Autodesk Inventor part; units mm, degrees
ref_plane "XZ Plane" through (0, 0, 0) normal (0, 1, 0) x (-1, 0, 0)
ref_plane "XY Plane" through (0, 0, 0) normal (0, 0, 1) x (1, 0, 0)
ref_plane "РабПлоскость1" through (0, 0, 0) normal (0, 0, 1) x (1, 0, 0)
sketch "Эскиз1" plane through (0, 0, 0) normal (0, 0, 1) x (1, 0, 0)
  circle A0 centre (72.7898, 20) radius 1.5 construction
  circle A1 centre (72.7898, -20) radius 1.5 construction
  line L0 (72.7898, 20) -> (72.7898, -20) construction
  circle A2 centre (72.7898, 0) radius 13.6
  circle A3 centre (72.7898, 20) radius 3.5
  circle A4 centre (72.7898, -20) radius 3.5
  line L1 (76.2898, 20) -> (69.2898, 20) construction
  line L2 (76.2898, -20) -> (69.2898, -20) construction
  line L3 (82.4064, 9.6167) -> (63.1731, -9.6167) construction
  line L4 (82.4064, -9.6167) -> (63.1731, 9.6167) construction
  arc A5 (76.2898, 20) -> (82.4064, 9.6167) centre (99.4251, 26.6354) ccw
  arc A6 (63.1731, 9.6167) -> (69.2898, 20) centre (46.1544, 26.6354) ccw
  arc A7 (69.2898, -20) -> (63.1731, -9.6167) centre (46.1544, -26.6354) ccw
  arc A8 (82.4064, -9.6167) -> (76.2898, -20) centre (99.4251, -26.6354) ccw
  circle A9 centre (72.7898, 0) radius 12.6
  point P0 (0, 0)
  point P1 (72.7898, 0)
  dimension "d0" = 27.2
  dimension "d3" = 7
  dimension "d4" = 45
  dimension "d5" = 25.2
extrude "Выдавливание1" add sketch "Эскиз1" along normal blind 40
hole "Отверстие1" at (72.7898, 20, 0) at (72.7898, -20, 0) direction (0, 0, 1) diameter 3.8 depth 6
sketch "Эскиз2" plane through (0, 0, 0) normal (0, 1, 0) x (-1, 0, 0)
  point P0 (0, 0)
ref_plane "РабПлоскость2" through (72.7898, -23.5, 40) normal (1, 0, 0) x (0, 1, 0)
properties part number "Крепление конденсатора"
Input: part model. Units: mm. Frame: model coordinates. A direction names the side the tool comes from. Round coordinates to 2 decimals unless told otherwise and drop trailing zeros. Order: outer loops, then holes, each group sorted by start corner. A loop starts at its lowest first (then second) coordinate and runs counter-clockwise, first axis right, second up.
1. Cut plane B-B, the plane x = 61.25. Output: boundary loops of the cut face in (y, z).
The answers:
outline: (-7.2, 0) - (-5.06, 0) - (-5.06, 40) - (-7.2, 40) - close; (5.06, 0) - (7.2, 0) - (7.2, 40) - (5.06, 40) - close
2. Cut plane C-C, the plane z = 37. Output: boundary loops of the cut face in (x, y), then the cut area to 3 significant figures.
The answers:
outline: (63.17, -9.62) arc R24.07 cw to (69.29, -20) arc R3.5 ccw to (76.29, -20) arc R24.07 cw to (82.41, -9.62) arc R13.6 ccw to (82.41, 9.62) arc R24.07 cw to (76.29, 20) arc R3.5 ccw to (69.29, 20) arc R24.07 cw to (63.17, 9.62) arc R13.6 ccw to start; hole circle Ø25.2 at (72.79, 0)
area: 263 mm2
3. Material intervals for line 1 (X direction, y = 20, z = 2); line 2 (Y direction, x = 73, z = 25); line 3 (Y direction, x = 82, z = 11.5), sorted ascending.
The answers:
line 1: x = 69.29 to 70.89, 74.69 to 76.29
line 2: y = -23.49 to -12.6, 12.6 to 23.49
line 3: y = -10.03 to -8.6, 8.6 to 10.03
4. Mould query, pull axis Y, two halves, no side actions, for faces 1 (the face through (84.429, 4.826, 19.72)), 2 (the face through (59.19, -0.15, 19.72)), 3 (the face through (72.9, -23.5, 19.7)). Classes: released by +Y, released by -Y, zero draft, split by the parting line, or undercut.
The answers:
face 1: undercut
face 2: split by the parting line
face 3: released by -Y
5. Pin query (flat end, axial travel): P1, Ø3, axis at x = 81.5, z = 24.5, coming from the -Y side; P2, Ø4, axis at y = -8.5, z = 32, coming from the +X side; P3, Ø2.5, axis at x = 72.79, y = -20, coming from the -Z side. Return the tip coordinate at first contact, or that it passes through.
The answers:
P1: stops at y = -12.42
P2: stops at x = 84.74
P3: stops at z = 6
6. Set-up query: faces 4 (the face through (66.935, 14.493, 19.72)), 5 (the face through (73, 20, 6)). Return all of +Z, -Z, +X, -X, +Y, -Y with unobstructed straight access to the full face (end or side cutting, diameter ignored); none if empty.
The answers:
face 4: +Z, -Z, -X, +Y
face 5: -Z
7. Cut plane D-D, the plane z = 4. Output: boundary loops of the cut face in (x, y).
The answers:
outline: (63.17, -9.62) arc R24.07 cw to (69.29, -20) arc R3.5 ccw to (76.29, -20) arc R24.07 cw to (82.41, -9.62) arc R13.6 ccw to (82.41, 9.62) arc R24.07 cw to (76.29, 20) arc R3.5 ccw to (69.29, 20) arc R24.07 cw to (63.17, 9.62) arc R13.6 ccw to start; hole circle Ø25.2 at (72.79, 0); hole circle Ø3.8 at (72.79, -20); hole circle Ø3.8 at (72.79, 20)
8. Cut plane A-A, the plane y = 0. Output: boundary loops of the cut face in (x, z).
The answers:
outline: (59.19, 0) - (60.19, 0) - (60.19, 40) - (59.19, 40) - close; (85.39, 0) - (86.39, 0) - (86.39, 40) - (85.39, 40) - close
